The listing builds one solid part. Answer for the finished solid, in the listing's coordinates (mm). Face numbers are marked on the shaded views. A direction names the side the tool comes from. Coordinates: 2 decimals unless noted, no trailing zeros. Write each loop counter-clockwise with the first axis right and the second up, starting at its lowest first coordinate (ties: lowest second). Pieces come first, ordered by that corner, then holes.
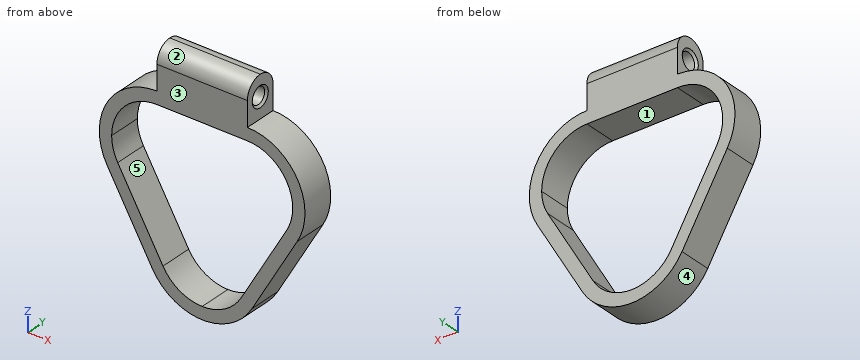
from build123d import *

# Parameters (mm, degrees)
F1_DEPTH       = 8
F2_DEPTH       = 10
F5_D           = 4
F5_DEPTH       = 12.7
F5_CSINK_D     = 5
F5_CSINK_ANGLE = 90
F5_TIP         = 1.2017212381
F6_D           = 4
F6_DEPTH       = 15
F6_CSINK_D     = 5
F6_CSINK_ANGLE = 90
F6_TIP         = 1.2017212381
F7_R           = 3.99999


# Not quite as in the source:
# - a fillet or chamfer is up to 0.001 mm smaller than in the source, because OpenCascade refuses the exact size


with BuildPart() as f1:
    # F0 (on Front) → F1 (new body)
    with BuildSketch(Plane.XZ):
        with BuildLine():
            ThreePointArc((0, 14), (-12.124355653, 7), (-12.124355653, -7))
            Line((-12.124355653, -7), (-1.124355653, -26.0525588833))
            ThreePointArc((-1.124355653, -26.0525588833), (11, -33.0525588833), (23.124355653, -26.0525588833))
            Line((23.124355653, -26.0525588833), (34.124355653, -7))
            ThreePointArc((34.124355653, -7), (34.124355653, 7), (22, 14))
            Line((22, 14), (0, 14))
        make_face()
        with BuildLine():
            ThreePointArc((-11, 0), (-7.7781745931, 7.7781745931), (0, 11))
            Line((0, 11), (11, 11))
            Line((11, 11), (22, 11))
            ThreePointArc((22, 11), (29.7781745931, 7.7781745931), (33, 0))
            ThreePointArc((33, 0), (32.6251840892, -2.8470094961), (31.5262794416, -5.5))
            Line((31.5262794416, -5.5), (20.5262794416, -24.5525588833))
            ThreePointArc((20.5262794416, -24.5525588833), (16.5, -28.5788383249), (11, -30.0525588833))
            ThreePointArc((11, -30.0525588833), (5.5, -28.5788383249), (1.4737205584, -24.5525588833))
            Line((1.4737205584, -24.5525588833), (-9.5262794416, -5.5))
            ThreePointArc((-9.5262794416, -5.5), (-10.6251840892, -2.8470094961), (-11, 0))
        make_face(mode=Mode.SUBTRACT)
    extrude(amount=F1_DEPTH)

    # F2 (add): a face of the model
    f2_faces = [f1.faces().sort_by_distance(p)[0] for p in [
        (11, -4, 14),
    ]]
    extrude(f2_faces, amount=F2_DEPTH)

    # F5
    with Locations(Plane.YZ.offset(22)):
        with Locations((-4, 19)):
            CounterSinkHole(F5_D / 2, F5_CSINK_D / 2, depth=F5_DEPTH, counter_sink_angle=F5_CSINK_ANGLE)
            with Locations((0, 0, -(F5_DEPTH + F5_TIP / 2))):  # 118° drill point
                Cone(0, F5_D / 2, F5_TIP, mode=Mode.SUBTRACT)

    # F6
    with Locations(Plane(origin=(0, 0, 0), x_dir=(0, -1, 0), z_dir=(-1, 0, 0))):
        with Locations((4, 19)):
            CounterSinkHole(F6_D / 2, F6_CSINK_D / 2, depth=F6_DEPTH, counter_sink_angle=F6_CSINK_ANGLE)
            with Locations((0, 0, -(F6_DEPTH + F6_TIP / 2))):  # 118° drill point
                Cone(0, F6_D / 2, F6_TIP, mode=Mode.SUBTRACT)

    # F7 (radius 4 in the source; OpenCascade refuses exactly that, so slightly less here)
    f7_edges = [f1.edges().sort_by_distance(p)[0] for p in [
        (11, 0, 24),
        (11, -8, 24),
    ]]
    fillet(f7_edges, radius=F7_R)


solid = f1.part
Q1. The part is cut by section C-C, the plane y = -5.25. State how many separate pieces and enclosed holes the cut face has, then the cut area to 3 significant figures.
Answers below:
separate pieces: 2
enclosed holes: 1
area: 580 mm2
Q2. Given pin 1 (1.5 mm diameter, centred on y = -6.5, z = -1.5, fed in from +X); pin 2 (4.5 mm diameter, centred on y = -4, z = 19, fed in from -X); pin 3 (2.5 mm diameter, centred on x = 14.5, y = -3.5, fed in from -Z), each flat-ended and moving along its own axis, determine where each tip first touches the part or whether it passes through.
Answers below:
pin 1: stops at x = 35.98
pin 2: stops at x = 0.25
pin 3: stops at z = -32.87
Q3. Find the intervals of material crossed by probe 1 along Y at (x, z) = (2.75, 19); probe 2 along Z at (x, y) = (3, -3.5); probe 3 along Z at (x, y) = (7.5, -4), in increasing order.
Answers below:
probe 1: y = -8 to -6, -2 to 0
probe 2: z = -30.54 to -26.6, 11 to 17.06, 20.94 to 23.97
probe 3: z = -32.61 to -29.48, 11 to 17, 21 to 24
Q4. The part is cut by section D-D, the plane z = 15. Write down the section's boundary in (x, y).
Answers below:
outline: (0, -8) - (22, -8) - (22, 0) - (0, 0) - close
Q5. Determine the mould class of the marked faces 1, 2 and 3 for opening direction Z: released by +Z, released by -Z, zero draft, split by the parting line, or undercut.
Answers below:
face 1: undercut
face 2: released by +Z
face 3: zero draft
Q6. The part is cut by section A-A, the plane x = 26. Write down the section's boundary in (y, z), then the cut area to 3 significant figures.
Answers below:
outline: (-8, -21.07) - (0, -21.07) - (0, -15.07) - (-8, -15.07) - close; (-8, 10.25) - (0, 10.25) - (0, 13.42) - (-8, 13.42) - close
area: 73.4 mm2
Q7. Which of the six approach directions +Z, -Z, +X, -X, +Y, -Y give full straight-line access (tool end or side, diameter ignored) to the marked faces 4 and 5?
Answers below:
face 4: -Z, +Y, -Y
face 5: +Y, -Y
Q8. The part is cut by section B-B, the plane z = 5.5. Write down the section's boundary in (x, y), then the cut area to 3 significant figures.
Answers below:
outline: (-12.87, -8) - (-9.53, -8) - (-9.53, 0) - (-12.87, 0) - close; (31.53, -8) - (34.87, -8) - (34.87, 0) - (31.53, 0) - close
area: 53.6 mm2
